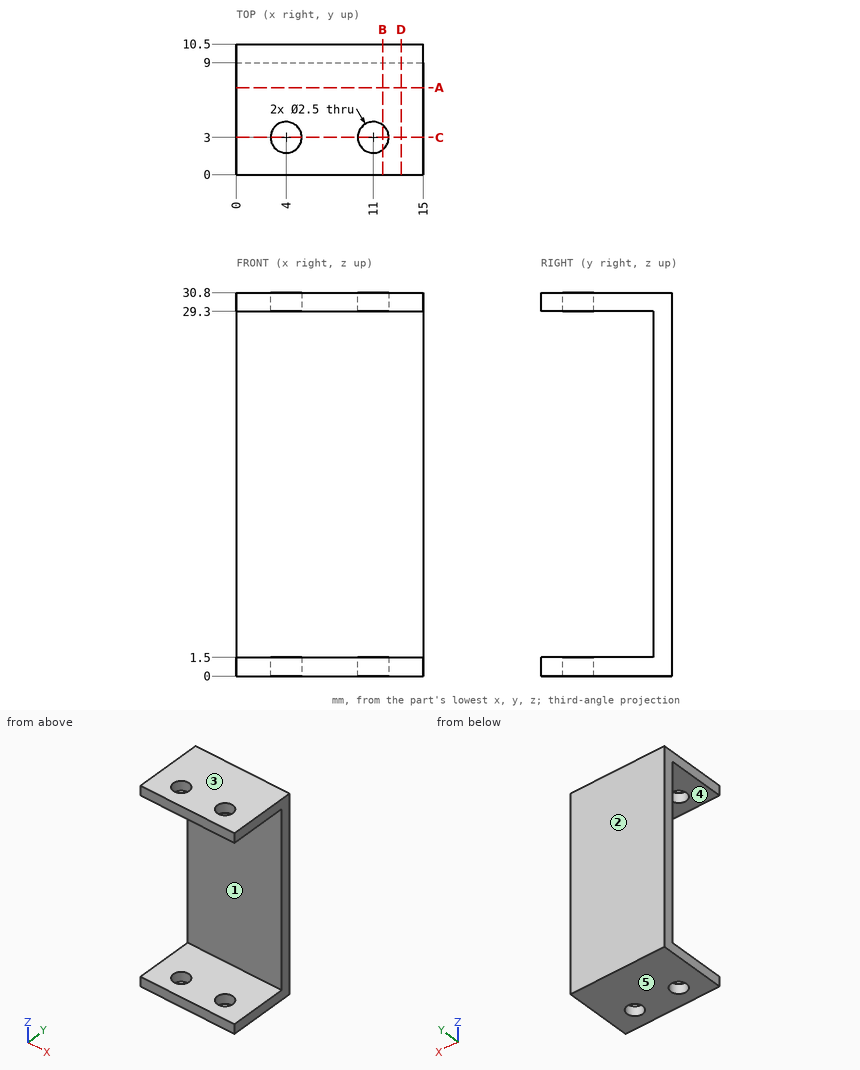
The drawing under review shows one solid part. Ordinate dimensions are in mm from its lowest x, y, z. A direction names the side the tool comes from. Round coordinates to 2 decimals unless told otherwise and drop trailing zeros. Write each loop counter-clockwise with the first axis right and the second up, starting at its lowest first coordinate (ties: lowest second). Pieces come first, ordered by that corner, then holes. Notation, with made-up numbers: (-18, 46) -> (5, 46) arc R13 cw to (5, 64) -> close; hole circle Ø3 at (39.5, 3.5). An arc over 180 degrees is marked (long way). One line per question, with ' | ' between items. Start each with the question number.
(1) For line 1 along Z through (x, y) = (5.5, 4); line 2 along Y through (x, z) = (11, 30); line 3 along Y through (x, z) = (6.75, 10), list the stretches that pass through material, from the lowest coordinate up. Write a range as from..to.
(2) Mouldability with a two-part tool opening along Z and no side actions: class the marked faces 3, 4 and 5 as released by +Z, released by -Z, zero draft, split by the parting line, or undercut.
(3) Tool access review of the marked faces 1 and 2: name each direction out of +Z, -Z, +X, -X, +Y, -Y from which nothing blocks a thin tool from reaching the whole face with its end or side.
(4) Add section B-B, the plane x = 11.75. Write out the cut boundary in (y, z), plus the area to 3 significant figures.
(5) Add section A-A, the plane y = 7. Write out the cut boundary in (x, z).
(6) Add section D-D, the plane x = 13.25. Write out the cut boundary in (y, z), plus the area to 3 significant figures.
(7) Insertion check: P1, Ø1.5, axis at x = 11, y = 3, coming from the +Z side; P2, Ø1, axis at x = 8.5, z = 9.5, coming from the -Y side. Each pin has a flat end and moves straight along its axis. Give the tip position at first contact, or say it passes through.
(8) Add section C-C, the plane y = 3. Write out the cut boundary in (x, z), plus the area to 3 significant figures.
Answer list:
1) line 1: 0..1.5, 29.3..30.8 | line 2: 0..1.75, 4.25..10.5 | line 3: 9..10.5
2) face 3: released by +Z | face 4: undercut | face 5: released by -Z
3) face 1: +X, -X, -Y | face 2: +Z, -Z, +X, -X, +Y
4) outline: (0, 0) -> (2, 0) -> (2, 1.5) -> (0, 1.5) -> close; (0, 29.3) -> (2, 29.3) -> (2, 30.8) -> (0, 30.8) -> close; (4, 0) -> (10.5, 0) -> (10.5, 30.8) -> (4, 30.8) -> (4, 29.3) -> (9, 29.3) -> (9, 1.5) -> (4, 1.5) -> close | area: 67.2 mm²
5) outline: (0, 0) -> (15, 0) -> (15, 1.5) -> (0, 1.5) -> close; (0, 29.3) -> (15, 29.3) -> (15, 30.8) -> (0, 30.8) -> close
6) outline: (0, 0) -> (10.5, 0) -> (10.5, 30.8) -> (0, 30.8) -> (0, 29.3) -> (9, 29.3) -> (9, 1.5) -> (0, 1.5) -> close | area: 73.2 mm²
7) P1: through | P2: y = 9
8) outline: (0, 0) -> (2.75, 0) -> (2.75, 1.5) -> (0, 1.5) -> close; (0, 29.3) -> (2.75, 29.3) -> (2.75, 30.8) -> (0, 30.8) -> close; (5.25, 0) -> (9.75, 0) -> (9.75, 1.5) -> (5.25, 1.5) -> close; (5.25, 29.3) -> (9.75, 29.3) -> (9.75, 30.8) -> (5.25, 30.8) -> close; (12.25, 0) -> (15, 0) -> (15, 1.5) -> (12.25, 1.5) -> close; (12.25, 29.3) -> (15, 29.3) -> (15, 30.8) -> (12.25, 30.8) -> close | area: 30.0 mm²
